Could you check a few things on this model? Use its own coordinates, in mm. Face numbers are marked on the shaded views. A direction names the side the tool comes from. Round coordinates to 2 decimals unless told otherwise and drop trailing zeros. Write each loop counter-clockwise with the first axis right and the second up, starting at its lowest first coordinate (ties: lowest second). Pieces come first, ordered by that corner, then holes. Notation, with made-up numbers: (-31, 70.25) -> (-6, 70.25) arc R26 ccw to (-6, 102.25) -> close; hole circle Ø4 at (10, 50). An arc over 180 degrees is marked (long way). One line per question, with ' | ' between items. Start each with the question number.
1. Imagine slicing it at A-A, the plane y = 0. List the corners of the cut face in (x, z) for me.
2. For the marked faces 4 and 5, which set-ups out of +Z, -Z, +X, -X, +Y, -Y let a thin tool reach every point of the face, with its end or its side?
3. For pin 1 Ø4 at (y, z) = (14, 36.5) entering from -X, with a flat end and sliding along its axis, tell me the tip position at first contact or that it passes through.
4. If I drill on line 1 along Z through (x, y) = (-4.5, 23.5); line 2 along Y through (x, z) = (0, 30); line 3 along Y through (x, z) = (3.5, 2), over which ranges is the centre line in solid material (lowest first)? Write a range as [from, to].
5. Thinking about a two-plate mould opening in X: for the marked faces 1, 2 and 3, which applies, released by +X, released by -X, zero draft, split by the parting line, or undercut?
6. Imagine slicing it at D-D, the plane x = -21.5. List the corners of the cut face in (y, z) for me.
7. Imagine slicing it at C-C, the plane z = 11. List the corners of the cut face in (x, y) for me, and give its area (3 significant figures).
from build123d import *

# Parameters (mm, degrees)
SKETCH1_R           = 16
SKETCH1_R_2         = 15
BOSS_EXTRUDE1_DEPTH = 50
SKETCH2_R           = 30
SKETCH2_R_2         = 15
BOSS_EXTRUDE2_DEPTH = 4


with BuildPart() as part:
    # Sketch1 → Boss-Extrude1 (new body)
    with BuildSketch(Plane.XY):
        Circle(SKETCH1_R)
        Circle(SKETCH1_R_2, mode=Mode.SUBTRACT)
    extrude(amount=BOSS_EXTRUDE1_DEPTH)

    # Sketch2 → Boss-Extrude2 (add)
    with BuildSketch(Plane.XY.offset(50)):
        Circle(SKETCH2_R)
        Circle(SKETCH2_R_2, mode=Mode.SUBTRACT)
    boss_extrude2 = extrude(amount=BOSS_EXTRUDE2_DEPTH)

    # Mirror1: Boss-Extrude2 across plane
    add(boss_extrude2.mirror(Plane(origin=(0, 0, 25), x_dir=(1, 0, 0), z_dir=(0, 0, -1))))


solid = part.part
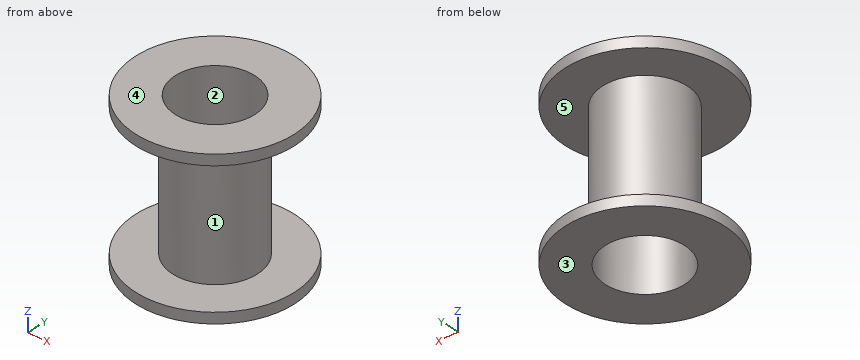
Geometry results:
1) outline: (-30, -4) -> (-15, -4) -> (-15, 54) -> (-30, 54) -> (-30, 50) -> (-16, 50) -> (-16, 0) -> (-30, 0) -> close; (15, -4) -> (30, -4) -> (30, 0) -> (16, 0) -> (16, 50) -> (30, 50) -> (30, 54) -> (15, 54) -> close
2) face 4: +Z, +X, -X, +Y, -Y | face 5: none
3) pin 1: stops at x = -10.58
4) line 1: z = [-4, 0], [50, 54] | line 2: y = [-16, -15], [15, 16] | line 3: y = [-15.61, -14.59], [14.59, 15.61]
5) face 1: split by the parting line | face 2: undercut | face 3: zero draft
6) outline: (-20.92, -4) -> (20.92, -4) -> (20.92, 0) -> (-20.92, 0) -> close; (-20.92, 50) -> (20.92, 50) -> (20.92, 54) -> (-20.92, 54) -> close
7) outline: circle Ø32 at (0, 0); hole circle Ø30 at (0, 0) | area: 97.4 mm2
